Autodesk Inventor part; units mm, degrees
ref_plane "YZ Plane" through (0, 0, 0) normal (1, 0, 0) x (0, 1, 0)
ref_plane "XZ Plane" through (0, 0, 0) normal (0, 1, 0) x (-1, 0, 0)
ref_plane "XY Plane" through (0, 0, 0) normal (0, 0, 1) x (1, 0, 0)
sketch "Sketch1" plane through (0, 0, 0) normal (0, 1, 0) x (-1, 0, 0)
  circle A0 centre (0, 0) radius 105
  dimension "d0" = 210
extrude "Extrusion1" add sketch "Sketch1" along normal blind 10
sketch "Sketch2" plane through (0, 10, 0) normal (0, 1, 0) x (1, 0, 0)
  circle A0 centre (0, 0) radius 2.5
  dimension "d3" = 5
extrude "Extrusion2" cut sketch "Sketch2" against normal blind 10
sketch "Sketch3" plane through (0, 10, 0) normal (0, 1, 0) x (1, 0, 0)
  circle A0 centre (0, 0) radius 2.5
  line L0 (0, 0) -> (0, -75)
  line L1 (0, -75) -> (-15, -75)
  circle A1 centre (-30, 0) radius 2.5
  circle A2 centre (-15, 0) radius 2.5
  circle A3 centre (0, 0) radius 2.5
  line L2 (15, 70.5) -> (15, 94.5)
  line L3 (0, 0) -> (29.6742, 0)
  line L4 (15, -70.5) -> (15, -94.5)
  circle A4 centre (-15, 70.5) radius 2.5
  circle A5 centre (0, 70.5) radius 2.5
  circle A6 centre (15, 70.5) radius 2.5
  circle A7 centre (-15, 94.5) radius 2.5
  circle A8 centre (0, 94.5) radius 2.5
  circle A9 centre (15, 94.5) radius 2.5
  circle A10 centre (-15, -70.5) radius 2.5
  circle A11 centre (0, -70.5) radius 2.5
  circle A12 centre (15, -70.5) radius 2.5
  circle A13 centre (-15, -94.5) radius 2.5
  circle A14 centre (0, -94.5) radius 2.5
  circle A15 centre (15, -94.5) radius 2.5
  dimension "d9" = 75
  dimension "d10" = 15
  dimension "d19" = 5
  dimension "d20" = 5
  dimension "d21" = 5
  dimension "d25" = 5
  dimension "d26" = 5
  dimension "d27" = 5
  dimension "d28" = 5
  dimension "d29" = 5
  dimension "d30" = 5
  dimension "d31" = 5
  dimension "d32" = 5
  dimension "d33" = 5
  dimension "d34" = 5
  dimension "d35" = 5
  dimension "d36" = 5
extrude "Extrusion3" cut sketch "Sketch3" against normal blind 10 contours A11 L0 | L0 A11 | A9 | A6 | A15 | A12 | A4 | A5 | A7 | A8 | A10 | A13 | A14
sketch "Sketch4" plane through (0, 10, 0) normal (0, 1, 0) x (1, 0, 0)
  circle A0 centre (-15, 94.5) radius 2
  circle A1 centre (0, 94.5) radius 2
  circle A2 centre (15, 94.5) radius 2
  circle A3 centre (15, 70.5) radius 2
  circle A4 centre (0, 70.5) radius 2
  circle A5 centre (-15, 70.5) radius 2
  circle A6 centre (15, -70.5) radius 2
  circle A7 centre (15, -94.5) radius 2
  circle A8 centre (0, -94.5) radius 2
  circle A9 centre (-15, -94.5) radius 2
  circle A10 centre (-15, -70.5) radius 2
  circle A11 centre (0, -70.5) radius 2
  line L0 (-22.4241, -99.4431) -> (24.1315, -99.4431)
  line L1 (24.1315, -99.4431) -> (24.1315, 99.2987)
  line L2 (24.1315, 99.2987) -> (-24.4086, 99.2987)
  line L3 (-24.4086, 99.2987) -> (-22.4241, -99.4431)
  point P0 (0, 0)
  dimension "d39" = 4
  dimension "d40" = 4
  dimension "d41" = 4
  dimension "d42" = 4
  dimension "d43" = 4
  dimension "d44" = 4
  dimension "d45" = 4
  dimension "d46" = 4
  dimension "d47" = 4
  dimension "d48" = 4
  dimension "d49" = 4
  dimension "d50" = 4
extrude "Extrusion4" add sketch "Sketch4" against normal blind 10
properties part number "Base do tripé"
The listing builds one solid part. Answer for the finished solid, in the listing's coordinates (mm). Give positions to 0.01 mm unless a question says otherwise; leave off trailing zeros. Order: outer loops, then holes, each group sorted by start corner. A loop starts at its lowest first (then second) coordinate and runs counter-clockwise, first axis right, second up. Notation, with made-up numbers: (40, 18.25) -> (61, 18.25) arc R6 cw to (61, 25.25) -> close; hole circle Ø9 at (72, -25.75). An arc over 180 degrees is marked (long way). Write each question's results on one line, items separated by ' | '.
Q1. Straight lines are drawn through the part: probe 1 along Z at (x, y) = (0, 5.5); probe 2 along X at (y, z) = (3.5, -94); probe 3 along X at (y, z) = (4.75, -76). For each, find the intervals that lie inside material, in ascending order. Write a range as from..to.
Checked values:
probe 1: z = -105..-96.5, -92.5..-72.5, -68.5..68.5, 72.5..92.5, 96.5..105 | probe 2: x = -46.79..-16.94, -13.06..-1.94, 1.94..13.06, 16.94..46.79 | probe 3: x = -72.45..72.45
Q2. The part is cut by section C-C, the plane x = 91. Give the vertices of the cut face in (y, z), and give its area (3 significant figures).
Checked values:
outline: (0, -52.38) -> (10, -52.38) -> (10, 52.38) -> (0, 52.38) -> close | area: 1,050 mm^2
Q3. The part is cut by section B-B, the plane z = 46. Give the vertices of the cut face in (x, y).
Checked values:
outline: (-94.39, 0) -> (94.39, 0) -> (94.39, 10) -> (-94.39, 10) -> close
Q4. Each of these flat-tipped pins is pushed along its axis until it touches: P1, Ø2, axis at x = -10, y = 4, coming from the +Z side; P2, Ø4, axis at x = 55, y = 5.5, coming from the -Z side; P3, Ø6, axis at x = 11, y = 6, coming from the +Z side. Where does it stop, or does it pass through?
Checked values:
P1: stops at z = 104.61 | P2: stops at z = -90.64 | P3: stops at z = 104.69
Q5. The part is cut by section A-A, the plane y = 5.5. State how many separate pieces and enclosed holes the cut face has, and give its area (3 significant figures).
Checked values:
separate pieces: 1 | enclosed holes: 12 | area: 34,500 mm^2
